The drawing under review shows one solid part. Ordinate dimensions are in mm from its lowest x, y, z. A direction names the side the tool comes from. Give positions to 0.01 mm unless a question says otherwise; leave off trailing zeros. Order: outer loops, then holes, each group sorted by start corner. A loop starts at its lowest first (then second) coordinate and runs counter-clockwise, first axis right, second up. Notation, with made-up numbers: (-1, -4) - (37, -4) arc R9 ccw to (37, 8) - close; hole circle Ø3 at (56.25, 59.5). An arc over 180 degrees is marked (long way). Use CSV: the item, a comma, the result in double quotes. Start each with the question number.
1. For pin 1 (12 mm diameter, centred on x = 45.5, y = 8, fed in from -Z); pin 2 (0.9 mm diameter, centred on x = 35, y = 24, fed in from +Z); pin 3 (9 mm diameter, centred on y = 15, z = 15.5, fed in from +X); pin 4 (2 mm diameter, centred on x = 38.5, z = 8, fed in from -Y), all flat-tipped, find the tip position at first contact; note any pin that passes through.
2. Take a section at C-C, the plane y = 7.5. State the section outline as (x, z) points.
3. Take a section at A-A, the plane z = 15.25. State the section outline as (x, y) points, then the cut area to 3 significant figures.
4. To check wall thickness, follow line 1 (Z direction, x = 30, y = 21.5); line 2 (X direction, y = 23, z = 19.25); line 3 (Z direction, x = 20, y = 18). State the ranges of each line that lie inside material, in increasing order. Write a range as [from, to].
5. Take a section at D-D, the plane x = 9.5. State the section outline as (y, z) points, then the cut area to 3 significant figures.
6. Take a section at B-B, the plane x = 26. State the section outline as (y, z) points.
7. Machinability: for the marked faces 1, 2, 3 and 4, which of the approach directions +Z, -Z, +X, -X, +Y, -Y give a long, thin tool a straight path to every point of the face, cutting with its end or side? Answer none if there is none.
8. Draft analysis for pull direction X (two halves, no side actions). For the marked faces 5, 6, 7 and 8, state which applies: released by +X, released by -X, zero draft, split by the parting line, or undercut.
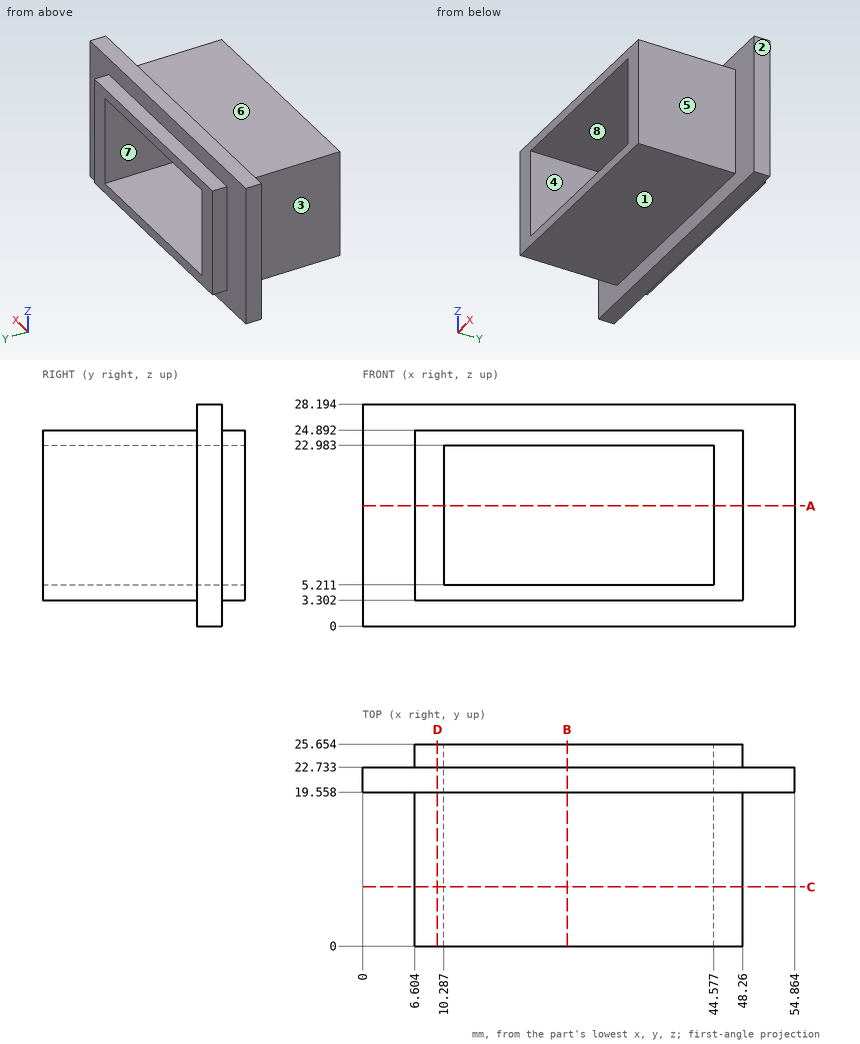
Determined:
1,pin 1,"stops at z = 3.3"
1,pin 2,"stops at z = 24.89"
1,pin 3,"stops at x = 48.26"
1,pin 4,"passes through"
2,outline,"(6.6, 3.3) - (48.26, 3.3) - (48.26, 24.89) - (6.6, 24.89) - close; hole (10.29, 5.21) - (44.58, 5.21) - (44.58, 22.98) - (10.29, 22.98) - close"
3,outline,"(0, 19.56) - (6.6, 19.56) - (6.6, 0) - (10.29, 0) - (10.29, 25.65) - (6.6, 25.65) - (6.6, 22.73) - (0, 22.73) - close; (44.58, 0) - (48.26, 0) - (48.26, 19.56) - (54.86, 19.56) - (54.86, 22.73) - (48.26, 22.73) - (48.26, 25.65) - (44.58, 25.65) - close"
3,area,"231 mm²"
4,line 1,"z = [0, 5.21], [22.98, 28.19]"
4,line 2,"x = [6.6, 10.29], [44.58, 48.26]"
4,line 3,"z = [3.3, 5.21], [22.98, 24.89]"
5,outline,"(0, 3.3) - (19.56, 3.3) - (19.56, 0) - (22.73, 0) - (22.73, 3.3) - (25.65, 3.3) - (25.65, 24.89) - (22.73, 24.89) - (22.73, 28.19) - (19.56, 28.19) - (19.56, 24.89) - (0, 24.89) - close"
5,area,"575 mm²"
6,outline,"(0, 3.3) - (19.56, 3.3) - (19.56, 0) - (22.73, 0) - (22.73, 3.3) - (25.65, 3.3) - (25.65, 5.21) - (0, 5.21) - close; (0, 22.98) - (25.65, 22.98) - (25.65, 24.89) - (22.73, 24.89) - (22.73, 28.19) - (19.56, 28.19) - (19.56, 24.89) - (0, 24.89) - close"
7,face 1,"-Z, +X, -X, -Y"
7,face 2,"+Z, -Z, +X, +Y, -Y"
7,face 3,"+Z, -Z, -X, -Y"
7,face 4,"+Y, -Y"
8,face 5,"released by +X"
8,face 6,"zero draft"
8,face 7,"undercut"
8,face 8,"undercut"
